The model under review builds one solid part; all positions refer to its coordinate system, in mm. Face numbers are marked on the shaded views. A direction names the side the tool comes from. Give positions to 0.01 mm unless a question says otherwise; leave off trailing zeros. Order: outer loops, then holes, each group sorted by start corner. A loop starts at its lowest first (then second) coordinate and runs counter-clockwise, first axis right, second up.
```python
from build123d import *

# Parameters (mm, degrees)
RESSALTO_EXTRUS_O1_DEPTH                = 3
BROCA_DE_ROSQUEAR_PARA_TARRAXA_DE_M31_D = 2.5
FURO_DE_DI_METRO_6_0_6_1_D              = 6
FURO_DE_DI_METRO_6_0_6_1_DEPTH          = 2
FURO_DE_DI_METRO_6_0_6_1_TIP            = 1.802581857
ESCAREADO_PARA_SFHCS_M31_D              = 3.4
ESCAREADO_PARA_SFHCS_M31_DEPTH          = 10
ESCAREADO_PARA_SFHCS_M31_CSINK_D        = 6.72
ESCAREADO_PARA_SFHCS_M31_CSINK_ANGLE    = 90
ESCAREADO_PARA_SFHCS_M31_TIP            = 1.021463052
ESBO_O10_R                              = 1.5
CORTE_EXTRUS_O1_DEPTH                   = 72.066727781
FILETE1_R                               = 2
FILETE2_R                               = 5
FURO_DE_DI_METRO_6_0_6_2_D              = 6
FURO_DE_DI_METRO_6_0_6_2_DEPTH          = 2
FURO_DE_DI_METRO_6_0_6_2_TIP            = 1.802581857


with BuildPart() as part:
    # Esboço1 → Ressalto-extrusão1 (new body)
    with BuildSketch(Plane.XY):
        with BuildLine():
            Line((-12, 30.768414179), (-12, 63))
            Line((-12, 63), (-27, 63))
            Line((-27, 63), (-27, 19.018288858))
            ThreePointArc((-27, 19.018288858), (-30.719082421, 12.125728279), (-32.710572622, 4.551236075))
            ThreePointArc((-32.710572622, 4.551236075), (-29.299973416, 0.038164719), (-24.786902061, 3.448763925))
            ThreePointArc((-24.786902061, 3.448763925), (-17.695825587, 17.695825587), (-3.448763925, 24.786902061))
            ThreePointArc((-3.448763925, 24.786902061), (-0.038164719, 29.299973416), (-4.551236075, 32.710572622))
            ThreePointArc((-4.551236075, 32.710572622), (-8.332397539, 31.957259931), (-12, 30.768414179))
        make_face()
    extrude(amount=RESSALTO_EXTRUS_O1_DEPTH)

    # Broca de rosquear para tarraxa de M31 (through all)
    with Locations(Plane.XY.offset(3)):
        with Locations((-28.748737342, 4), (-4, 28.748737342)):
            Hole(BROCA_DE_ROSQUEAR_PARA_TARRAXA_DE_M31_D / 2)

    # Furo de diâmetro Ø6.0 (6)1
    with Locations(Plane(origin=(0, 0, 0), x_dir=(-1, 0, 0), z_dir=(0, 0, -1))):
        with Locations((28.748737342, 4), (4, 28.748737342)):
            Hole(FURO_DE_DI_METRO_6_0_6_1_D / 2, depth=FURO_DE_DI_METRO_6_0_6_1_DEPTH)
            with Locations((0, 0, -(FURO_DE_DI_METRO_6_0_6_1_DEPTH + FURO_DE_DI_METRO_6_0_6_1_TIP / 2))):  # 118° drill point
                Cone(0, FURO_DE_DI_METRO_6_0_6_1_D / 2, FURO_DE_DI_METRO_6_0_6_1_TIP, mode=Mode.SUBTRACT)

    # Escareado para SFHCS M31
    with Locations(Plane(origin=(0, 0, 0), x_dir=(-1, 0, 0), z_dir=(0, 0, -1))):
        with Locations((15, 60.5), (24, 60.5)):
            CounterSinkHole(ESCAREADO_PARA_SFHCS_M31_D / 2, ESCAREADO_PARA_SFHCS_M31_CSINK_D / 2, depth=ESCAREADO_PARA_SFHCS_M31_DEPTH, counter_sink_angle=ESCAREADO_PARA_SFHCS_M31_CSINK_ANGLE)
            with Locations((0, 0, -(ESCAREADO_PARA_SFHCS_M31_DEPTH + ESCAREADO_PARA_SFHCS_M31_TIP / 2))):  # 118° drill point
                Cone(0, ESCAREADO_PARA_SFHCS_M31_D / 2, ESCAREADO_PARA_SFHCS_M31_TIP, mode=Mode.SUBTRACT)

    # Esboço10 → Corte-extrusão1 (cut, through all)
    with BuildSketch(Plane(origin=(0, 0, 0), x_dir=(-1, 0, 0), z_dir=(0, 0, -1))):
        with Locations((17.498454448, 28.544464197)):
            Circle(ESBO_O10_R)
        with BuildLine():
            Line((23.5, 45.518288858), (27, 45.518288858))
            Line((27, 45.518288858), (27, 38.518288858))
            Line((27, 38.518288858), (23.5, 38.518288858))
            ThreePointArc((23.5, 38.518288858), (20, 42.018288858), (23.5, 45.518288858))
        make_face()
    extrude(amount=-CORTE_EXTRUS_O1_DEPTH, mode=Mode.SUBTRACT)

    # Filete1
    filete1_edges = [part.edges().sort_by_distance(p)[0] for p in [
        (-27, 45.518288858, 1.5),
        (-27, 38.518288858, 1.5),
    ]]
    fillet(filete1_edges, radius=FILETE1_R)

    # Filete2
    filete2_edges = [part.edges().sort_by_distance(p)[0] for p in [
        (-27, 19.018288858, 1.5),
        (-12, 30.768414179, 1.5),
    ]]
    fillet(filete2_edges, radius=FILETE2_R)

    # Furo de diâmetro Ø6.0 (6)2
    with Locations(Plane.XY.offset(3)):
        with Locations((-17.498454448, 28.544464197)):
            Hole(FURO_DE_DI_METRO_6_0_6_2_D / 2, depth=FURO_DE_DI_METRO_6_0_6_2_DEPTH)
            with Locations((0, 0, -(FURO_DE_DI_METRO_6_0_6_2_DEPTH + FURO_DE_DI_METRO_6_0_6_2_TIP / 2))):  # 118° drill point
                Cone(0, FURO_DE_DI_METRO_6_0_6_2_D / 2, FURO_DE_DI_METRO_6_0_6_2_TIP, mode=Mode.SUBTRACT)


solid = part.part
```
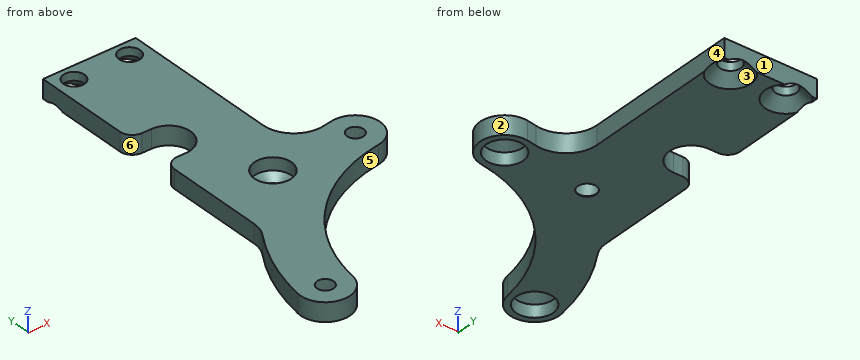
1. Take a section at B-B (y = 44). Write out the cut boundary in (x, z), and give its area (3 significant figures).
2. Draft analysis for pull direction Y (two halves, no side actions). For the marked faces 1, 2 and 3, state which applies: pulls with the +Y half, pulls with the -Y half, needs draft (parallel to the pull), parting line crosses it, or undercut.
3. Take a section at C-C (y = 14). Write out the cut boundary in (x, z), and give its area (3 significant figures).
4. To check wall thickness, follow line 1 (Y direction, x = -16, z = 1.4); line 2 (Y direction, x = -17, z = 1); line 3 (Y direction, x = -22, z = 2.5). State the ranges of each line that lie inside material, in increasing order.
5. For the marked faces 4, 5 and 6, list the 3-axis set-ups (+Z, -Z, +X, -X, +Y, -Y) from which the entire face can be reached by the end or side of a thin tool; tool diameter is ignored.
6. Take a section at A-A (z = 2.5). Write out the cut boundary in (x, y).
7. Insertion check: pin 1 (1.5 mm diameter, centred on y = 48.5, z = 1.5, fed in from -X); pin 2 (2.5 mm diameter, centred on x = -17.5, y = 28.54, fed in from -Z) (3 decimals); pin 3 (1.5 mm diameter, centred on y = 52, z = 1.5, fed in from +X); pin 4 (1.5 mm diameter, centred on y = 32, z = 2.5, fed in from +X). Each pin has a flat end and moves straight along its axis. Give the tip position at first contact, or say it passes through.
Answer:
1. outline: (-20.62, 0) - (-12, 0) - (-12, 3) - (-20.62, 3) - close
1. area: 25.8 mm2
2. face 1: pulls with the +Y half
2. face 2: parting line crosses it
2. face 3: undercut
3. outline: (-29.91, 0) - (-20.74, 0) - (-20.74, 3) - (-29.91, 3) - close
3. area: 27.5 mm2
4. line 1: y = 19.24 to 25.95, 31.14 to 58.81, 62.19 to 63
4. line 2: y = 18.37 to 25.59, 31.5 to 59.25, 61.75 to 63
4. line 3: y = 11.93 to 38.86, 45.18 to 63
5. face 4: +Z, -Z, +X, +Y
5. face 5: +Z, -Z, +X, -Y
5. face 6: +Z, -Z, -X
6. outline: (-32.71, 4.55) arc R4 ccw to (-24.79, 3.45) arc R25.03 cw to (-3.45, 24.79) arc R4 ccw to (-4.55, 32.71) arc R33.03 ccw to (-6.08, 32.46) arc R5 cw to (-12, 37.38) - (-12, 63) - (-27, 63) - (-27, 47.52) arc R2 ccw to (-25, 45.52) - (-23.5, 45.52) arc R3.5 cw to (-23.5, 38.52) - (-25, 38.52) arc R2 ccw to (-27, 36.52) - (-27, 20.54) arc R5 cw to (-27.79, 17.84) arc R33.03 ccw to start; hole circle Ø4.34 at (-28.75, 4); hole circle Ø3.4 at (-24, 60.5); hole circle Ø6 at (-17.5, 28.54); hole circle Ø3.4 at (-15, 60.5); hole circle Ø4.34 at (-4, 28.75)
7. pin 1: stops at x = -27
7. pin 2: passes through
7. pin 3: stops at x = -12
7. pin 4: stops at x = -0.88
